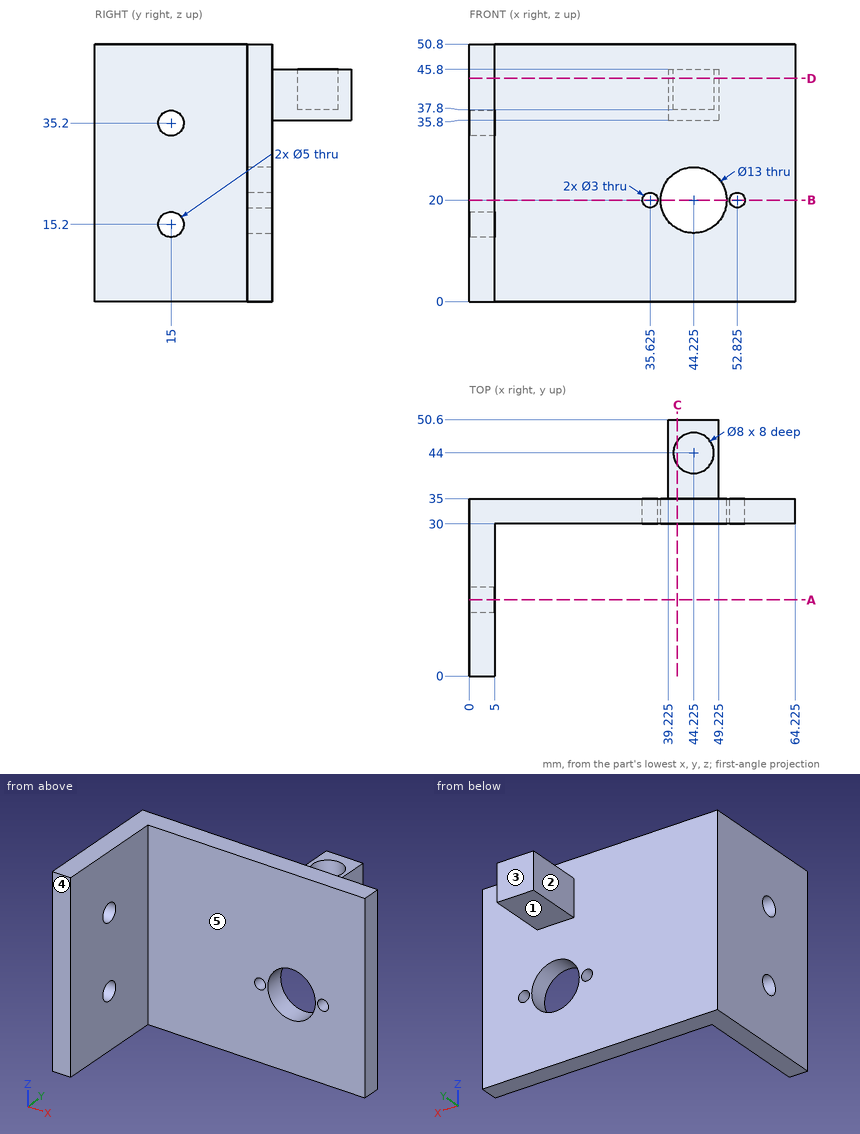
Verification items for this drawing (mm, ordinates from the low corner). A direction names the side the tool comes from. Round coordinates to 2 decimals unless told otherwise and drop trailing zeros. Loops run counter-clockwise (first coordinate to the right, second up) from the corner with the lowest first, then second, coordinate; pieces in that order, holes last. Notation, with made-up numbers: (76, -12) - (116, -12) arc R26 cw to (116, 2) - close; hole circle Ø2 at (17, 46). An arc over 180 degrees is marked (long way). Answer as CSV lines item,"result". Start each with the question number.
Item 1: Section check A-A (y = 15). Record the boundary of the cut face in (x, z).
Item 2: Section check D-D (z = 44). Record the boundary of the cut face in (x, y) (3 decimals), and give its area (3 significant figures).
Item 3: Depth check by flat-ended pin: P1, Ø10, axis at x = 48.5, z = 11, coming from the +Y side; P2, Ø7, axis at x = 44.225, y = 44, coming from the -Z side; P3, Ø24, axis at y = 20.5, z = 14, coming from the +X side (3 decimals); P4, Ø5, axis at y = 43.5, z = 42.5, coming from the -X side (3 decimals). Enter the tip coordinate at first touch or a pass-through.
Item 4: Scan lines: line 1 (X direction, y = 33.15, z = 20) (3 decimals); line 2 (Y direction, x = 1, z = 35); line 3 (Y direction, x = 3.5, z = 20). Record each from-to range of solid material in increasing order. Write a range as [from, to].
Item 5: Section check B-B (z = 20). Record the boundary of the cut face in (x, y) (3 decimals).
Item 6: Section check C-C (x = 41). Record the boundary of the cut face in (y, z), and give its area (3 significant figures).
Item 7: Set-up check for the marked faces 1, 2, 3, 4 and 5: record each of +Z, -Z, +X, -X, +Y, -Y from which the full face is reachable in a straight line by a thin tool's end or side.
Report:
1,outline,"(0, 0) - (5, 0) - (5, 12.7) - (0, 12.7) - close; (0, 17.7) - (5, 17.7) - (5, 32.7) - (0, 32.7) - close; (0, 37.7) - (5, 37.7) - (5, 50.8) - (0, 50.8) - close"
2,outline,"(0, 0) - (5, 0) - (5, 30) - (64.225, 30) - (64.225, 35) - (49.225, 35) - (49.225, 50.6) - (39.225, 50.6) - (39.225, 35) - (0, 35) - close; hole circle Ø8 at (44.225, 44)"
2,area,"577 mm2"
3,P1,"stops at y = 35"
3,P2,"stops at z = 35.8"
3,P3,"stops at x = 64.225"
3,P4,"stops at x = 39.225"
4,line 1,"x = [0, 34.125], [37.125, 37.725], [50.725, 51.325], [54.325, 64.225]"
4,line 2,"y = [0, 12.51], [17.49, 35]"
4,line 3,"y = [0, 35]"
5,outline,"(0, 0) - (5, 0) - (5, 30) - (34.125, 30) - (34.125, 35) - (0, 35) - close; (37.125, 30) - (37.725, 30) - (37.725, 35) - (37.125, 35) - close; (50.725, 30) - (51.325, 30) - (51.325, 35) - (50.725, 35) - close; (54.325, 30) - (64.225, 30) - (64.225, 35) - (54.325, 35) - close"
6,outline,"(30, 0) - (35, 0) - (35, 14.36) - (30, 14.36) - close; (30, 25.64) - (35, 25.64) - (35, 35.8) - (50.6, 35.8) - (50.6, 45.8) - (46.37, 45.8) - (46.37, 37.8) - (41.63, 37.8) - (41.63, 45.8) - (35, 45.8) - (35, 50.8) - (30, 50.8) - close"
6,area,"316 mm2"
7,face 1,"-Z, +X, -X, +Y"
7,face 2,"+Z, -Z, -X, +Y"
7,face 3,"+Z, -Z, +X, -X, +Y"
7,face 4,"+Z, -Z, +X, -X, -Y"
7,face 5,"+Z, -Z, +X, -Y"
